Model file for the job. Use its own axes, mm. A direction names the side the tool comes from. Coordinates: 2 decimals unless noted, no trailing zeros. Order: outer loops, then holes, each group sorted by start corner. A loop starts at its lowest first (then second) coordinate and runs counter-clockwise, first axis right, second up. Notation, with made-up numbers: M -4,34 L 49,34 A22 ccw 49,60 Z; hole C 2.5,57 d9. An arc over 180 degrees is marked long. Return JSON: item names as keys, results as strings.
```python
from build123d import *

# Parameters (mm, degrees)
F0_R          = 2
F1_DEPTH      = 0.5
F2_DEPTH      = 1.5
F3_DEPTH      = 4.5
F5_R          = 0.75
F6_DEPTH      = 22
F6_DEPTH_BACK = 1.8118981114


# Not quite as in the source:
# - an extrude ends at something that could not be found from the text; its depth is read off the source's solid
# - a feature names something its author has since deleted; it is built from what else it names


with BuildPart() as f1:
    # F0 (on Top) → F1 (new body)
    with BuildSketch(Plane.XY):
        with BuildLine():
            ThreePointArc((3, -1.8027756377), (3.3726843908, -0.9354143467), (3.5, 0))
            ThreePointArc((3.5, 0), (2.4748737342, 2.4748737342), (0, 3.5))
            ThreePointArc((0, 3.5), (-0.9354143467, 3.3726843908), (-1.8027756377, 3))
            Line((-1.8027756377, 3), (0, 3))
            ThreePointArc((0, 3), (2.1213203436, 2.1213203436), (3, 0))
            Line((3, 0), (3, -1.8027756377))
        make_face()
        with BuildLine():
            ThreePointArc((-1.8027756377, 3), (-0.9354143467, 3.3726843908), (0, 3.5))
            Line((0, 3.5), (-2.8192741549, 3.5))
            Line((-2.8192741549, 3.5), (-2.8192741549, 3))
            Line((-2.8192741549, 3), (-1.8027756377, 3))
        make_face()
        with BuildLine():
            Line((3.5, -7.1381019886), (3.5, -6.5766632877))
            ThreePointArc((3.5, -6.5766632877), (3.2522630595, -6.7026326911), (3, -6.8192741549))
            ThreePointArc((3, -6.8192741549), (0.7871839081, -7.4082954514), (-1.5, -7.2974310548))
            Line((-1.5, -7.2974310548), (-1.5, -7.8072082078))
            ThreePointArc((-1.5, -7.8072082078), (1.0544789155, -7.8797572435), (3.5, -7.1381019886))
        make_face()
        with BuildLine():
            Line((3.5, -6.5766632877), (3.5, 0))
            ThreePointArc((3.5, 0), (3.3726843908, -0.9354143467), (3, -1.8027756377))
            Line((3, -1.8027756377), (3, -6.8192741549))
            ThreePointArc((3, -6.8192741549), (3.2522630595, -6.7026326911), (3.5, -6.5766632877))
        make_face()
        with BuildLine():
            Line((3, -6.8192741549), (3, -1.8027756377))
            ThreePointArc((3, -1.8027756377), (-2.4748737342, -2.4748737342), (-1.8027756377, 3))
            Line((-1.8027756377, 3), (-2.8192741549, 3))
            Line((-2.8192741549, 3), (-6.8192741549, 3))
            ThreePointArc((-6.8192741549, 3), (-6.619052213, -3.4191589319), (-1.5, -7.2974310548))
            ThreePointArc((-1.5, -7.2974310548), (0.7871839081, -7.4082954514), (3, -6.8192741549))
        make_face()
        with BuildLine():
            ThreePointArc((-1.8027756377, 3), (-2.4748737342, -2.4748737342), (3, -1.8027756377))
            Line((3, -1.8027756377), (3, 0))
            ThreePointArc((3, 0), (-2.1213203436, -2.1213203436), (0, 3))
            Line((0, 3), (-1.8027756377, 3))
        make_face()
        with BuildLine():
            ThreePointArc((0, 3), (-2.1213203436, -2.1213203436), (3, 0))
            ThreePointArc((3, 0), (2.1213203436, 2.1213203436), (0, 3))
        make_face()
        Circle(F0_R, mode=Mode.SUBTRACT)
    extrude(amount=F1_DEPTH)

    # F0 (on Top) → F2 (join)
    with BuildSketch(Plane.XY):
        with BuildLine():
            Line((3.5, -7.1381019886), (3.5, -6.5766632877))
            ThreePointArc((3.5, -6.5766632877), (3.2522630595, -6.7026326911), (3, -6.8192741549))
            ThreePointArc((3, -6.8192741549), (0.7871839081, -7.4082954514), (-1.5, -7.2974310548))
            Line((-1.5, -7.2974310548), (-1.5, -7.8072082078))
            ThreePointArc((-1.5, -7.8072082078), (1.0544789155, -7.8797572435), (3.5, -7.1381019886))
        make_face()
        with BuildLine():
            Line((3.5, -6.5766632877), (3.5, 0))
            ThreePointArc((3.5, 0), (3.3726843908, -0.9354143467), (3, -1.8027756377))
            Line((3, -1.8027756377), (3, -6.8192741549))
            ThreePointArc((3, -6.8192741549), (3.2522630595, -6.7026326911), (3.5, -6.5766632877))
        make_face()
        with BuildLine():
            ThreePointArc((3, -1.8027756377), (3.3726843908, -0.9354143467), (3.5, 0))
            ThreePointArc((3.5, 0), (2.4748737342, 2.4748737342), (0, 3.5))
            ThreePointArc((0, 3.5), (-0.9354143467, 3.3726843908), (-1.8027756377, 3))
            Line((-1.8027756377, 3), (0, 3))
            ThreePointArc((0, 3), (2.1213203436, 2.1213203436), (3, 0))
            Line((3, 0), (3, -1.8027756377))
        make_face()
        with BuildLine():
            ThreePointArc((-1.8027756377, 3), (-0.9354143467, 3.3726843908), (0, 3.5))
            Line((0, 3.5), (-2.8192741549, 3.5))
            Line((-2.8192741549, 3.5), (-2.8192741549, 3))
            Line((-2.8192741549, 3), (-1.8027756377, 3))
        make_face()
        with BuildLine():
            Line((-2.8192741549, 3), (-2.8192741549, 3.5))
            Line((-2.8192741549, 3.5), (-6.5766632877, 3.5))
            ThreePointArc((-6.5766632877, 3.5), (-6.7026326911, 3.2522630595), (-6.8192741549, 3))
            Line((-6.8192741549, 3), (-2.8192741549, 3))
        make_face()
        with BuildLine():
            ThreePointArc((-6.8192741549, 3), (-6.7026326911, 3.2522630595), (-6.5766632877, 3.5))
            Line((-6.5766632877, 3.5), (-7.1381019886, 3.5))
            ThreePointArc((-7.1381019886, 3.5), (-7.114593513, -3.5475426911), (-1.5, -7.8072082078))
            Line((-1.5, -7.8072082078), (-1.5, -7.2974310548))
            ThreePointArc((-1.5, -7.2974310548), (-6.619052213, -3.4191589319), (-6.8192741549, 3))
        make_face()
    extrude(amount=F2_DEPTH)

    # F0 (on Top) → F3 (join)
    with BuildSketch(Plane.XY):
        with BuildLine():
            ThreePointArc((-6.8192741549, 3), (-6.7026326911, 3.2522630595), (-6.5766632877, 3.5))
            Line((-6.5766632877, 3.5), (-7.1381019886, 3.5))
            ThreePointArc((-7.1381019886, 3.5), (-7.114593513, -3.5475426911), (-1.5, -7.8072082078))
            Line((-1.5, -7.8072082078), (-1.5, -7.2974310548))
            ThreePointArc((-1.5, -7.2974310548), (-6.619052213, -3.4191589319), (-6.8192741549, 3))
        make_face()
        with BuildLine():
            Line((-2.8192741549, 3), (-2.8192741549, 3.5))
            Line((-2.8192741549, 3.5), (-6.5766632877, 3.5))
            ThreePointArc((-6.5766632877, 3.5), (-6.7026326911, 3.2522630595), (-6.8192741549, 3))
            Line((-6.8192741549, 3), (-2.8192741549, 3))
        make_face()
    extrude(amount=F3_DEPTH)

    # F5 (on plane+point) → F6 (cut, two sides)
    with BuildSketch(Plane.YZ.offset(-7.1381019886)) as f6_sk:
        with BuildLine():
            ThreePointArc((2.75, 3.5), (2, 4.25), (1.25, 3.5))
            ThreePointArc((1.25, 3.5), (2, 2.75), (2.75, 3.5))
        make_face()
        with BuildLine():
            Line((0, 3.5), (0, 2.75))
            ThreePointArc((0, 2.75), (0.5303300859, 2.9696699141), (0.75, 3.5))
            Line((0.75, 3.5), (0, 3.5))
        make_face()
        with BuildLine():
            Line((-0.75, 3.5), (0, 3.5))
            Line((0, 3.5), (0.75, 3.5))
            ThreePointArc((0.75, 3.5), (0, 4.25), (-0.75, 3.5))
        make_face()
        with BuildLine():
            ThreePointArc((-0.75, 3.5), (-0.5303300859, 2.9696699141), (0, 2.75))
            Line((0, 2.75), (0, 3.5))
            Line((0, 3.5), (-0.75, 3.5))
        make_face()
        with Locations((-2, 3.5)):
            Circle(F5_R)
    extrude(amount=F6_DEPTH, mode=Mode.SUBTRACT)
    extrude(f6_sk.sketch, amount=-F6_DEPTH_BACK, mode=Mode.SUBTRACT)


solid = f1.part
```
Item 1: Saw through at A-A (z = 3.9). Write the cut outline in (x, y).
Check result:
{"outline": "M -7.92,-0.63 A7.95 ccw -7.83,-1.37 L -7.32,-1.37 A7.45 cw -7.42,-0.63 Z; M -7.92,0.63 L -7.42,0.63 A7.45 cw -7.32,1.37 L -7.83,1.37 A7.95 ccw Z; M -7.5,-2.63 A7.95 ccw -1.5,-7.81 L -1.5,-7.3 A7.45 cw -6.97,-2.63 Z; M -7.5,2.63 L -6.97,2.63 A7.45 cw -6.82,3 L -2.82,3 L -2.82,3.5 L -7.14,3.5 A7.95 ccw Z"}
Item 2: Wall check: line 1 (Y direction, x = -7.6, z = 3.5); line 2 (Z direction, x = -7.45, y = -2); line 3 (X direction, y = 0, z = 1.85). Give the ranges that are in metal, low to high.
Check result:
{"line 1": "y = -1.25 to -0.75, 0.75 to 1.25", "line 2": "z = 0 to 2.75, 4.25 to 4.5", "line 3": "x = -7.95 to -7.45"}
Item 3: Saw through at B-B (x = -0.5). Write the cut outline in (y, z).
Check result:
{"outline": "M -7.93,0 L -1.94,0 L -1.94,0.5 L -7.43,0.5 L -7.43,1.5 L -7.93,1.5 Z; M 1.94,0 L 3.5,0 L 3.5,1.5 L 3,1.5 L 3,0.5 L 1.94,0.5 Z"}
Item 4: Pull direction Y, two halves, no side cores. Call faces 1 (the cylindrical face through (2.1, 2.14, 0.99)), 2 (the flat face through (-2, -2, 0)), 3 (the cylindrical face through (-5.72, -5.52, 1.72)): +Y half, -Y half, draft (parallel to the pull), parting line (faces both ways), or undercut.
Check result:
{"face 1": "undercut", "face 2": "draft", "face 3": "parting line"}
Item 5: Saw through at D-D (x = -5.75). Write the cut outline in (y, z), and give its area (3 significant figures).
Check result:
{"outline": "M -5.49,0 L 3.5,0 L 3.5,4.5 L 3,4.5 L 3,0.5 L -4.74,0.5 L -4.74,4.5 L -5.49,4.5 Z", "area": "9.51 mm2"}
Item 6: Saw through at C-C (z = 1.05). Write the cut outline in (x, y), and give its area (3 significant figures).
Check result:
{"outline": "M -7.14,3.5 A7.95 ccw 3.5,-7.14 L 3.5,0 A3.5 ccw 0,3.5 Z; hole M -6.82,3 A7.45 ccw 3,-6.82 L 3,0 A3 ccw 0,3 Z", "area": "18.9 mm2"}
Item 7: 3-axis set-ups, long thin cutter, end or side, ignore diameter. For faces 4 (the cylindrical face through (-0.434, -1.952, 0.246)), 5 (the flat face through (3, -3, 1)): which of +Z, -Z, +X, -X, +Y, -Y reach the whole face in a straight line?
Check result:
{"face 4": "+Z, -Z", "face 5": "+Z"}
Item 8: Drop flat-ended pins along their axis: pin 1 Ø1 at (y, z) = (-5, 2.5) entering from +X; pin 2 Ø3 at (x, y) = (-0.5, 0.5) entering from +Z; pin 3 Ø1.5 at (x, z) = (1.5, 1.5) entering from +Y. Give the stop position or say it passes through.
Check result:
{"pin 1": "stops at x = -5.03", "pin 2": "stops at z = 0.5", "pin 3": "stops at y = 3.42"}
